Can you work these out from the drawing? Everything is in mm from the part's minimum corner. Give positions to 0.01 mm unless a question says otherwise; leave off trailing zeros. Write each loop counter-clockwise with the first axis right and the second up, starting at its lowest first coordinate (ties: lowest second). Pieces come first, ordered by that corner, then holes. Notation, with made-up numbers: (-14, 73) - (10, 73) arc R21 ccw to (10, 111) - close; hole circle Ø2 at (18, 31). An arc over 180 degrees is marked (long way). Use a Markdown table: item, result.
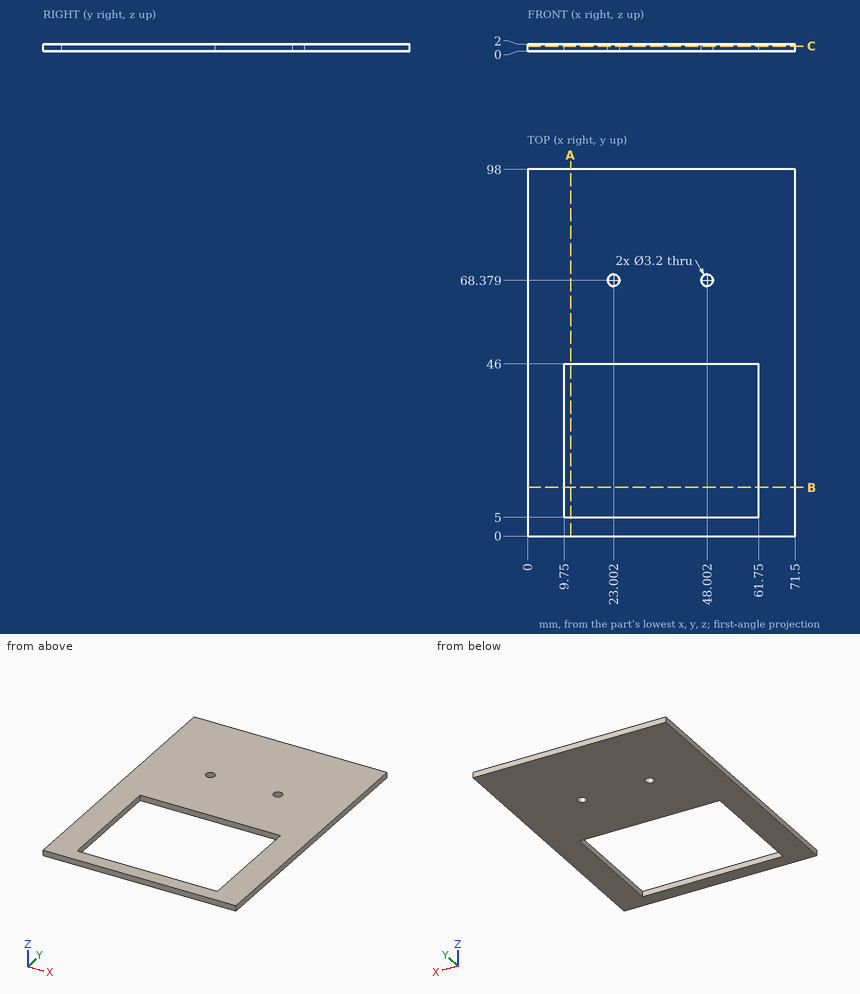
Item 1: If we section it at B-B, the plane y = 13: Write out the boundary of the cut face in (x, z), plus the area to 3 significant figures.
Values:
| item | result |
|---|---|
| outline | (0, 0) - (9.75, 0) - (9.75, 2) - (0, 2) - close; (61.75, 0) - (71.5, 0) - (71.5, 2) - (61.75, 2) - close |
| area | 39.0 mm2 |
Item 2: I need wall thicknesses on line 1 along Y through (x, z) = (25, 1.05); line 2 along Y through (x, z) = (22, 0.6) (1 decimal); line 3 along X through (y, z) = (24.5, 0.65). Which ranges of each line are inside material? Lowest first, please. Write a range as [from, to].
Values:
| item | result |
|---|---|
| line 1 | y = [0, 5], [46, 98] |
| line 2 | y = [0, 5], [46, 67.1], [69.6, 98] |
| line 3 | x = [0, 9.75], [61.75, 71.5] |
Item 3: Will these pins go through, and if not, where does the flat tip stop? pin 1 Ø3 at (x, y) = (48, 68.38) entering from +Z; pin 2 Ø4 at (x, y) = (64, 49) entering from -Z.
Values:
| item | result |
|---|---|
| pin 1 | passes through |
| pin 2 | stops at z = 0 |
Item 4: If we section it at A-A, the plane x = 11.5: Write out the boundary of the cut face in (y, z).
Values:
| item | result |
|---|---|
| outline | (0, 0) - (5, 0) - (5, 2) - (0, 2) - close; (46, 0) - (98, 0) - (98, 2) - (46, 2) - close |
Item 5: If we section it at C-C, the plane z = 1.4: Write out the boundary of the cut face in (x, y), plus the area to 3 significant figures.
Values:
| item | result |
|---|---|
| outline | (0, 0) - (71.5, 0) - (71.5, 98) - (0, 98) - close; hole (9.75, 5) - (61.75, 5) - (61.75, 46) - (9.75, 46) - close; hole circle Ø3.2 at (23, 68.38); hole circle Ø3.2 at (48, 68.38) |
| area | 4,860 mm2 |
